Geometry: final body of the model. Coordinates: model frame, mm. Face numbers are marked on the shaded views. A direction names the side the tool comes from. Coordinates: 2 decimals unless noted, no trailing zeros. Write each loop counter-clockwise with the first axis right and the second up, starting at its lowest first coordinate (ties: lowest second). Pieces come first, ordered by that corner, then holes. Notation, with made-up numbers: M -34.75,48.25 L -30.75,48.25 A31 ccw -30.75,78.25 Z; hole C -1.75,17 d1. An arc over 180 degrees is marked long. Write item = value, one per line. Start each with the question number.
Item 1: Reachability of the marked faces 1 and 2 from +Z, -Z, +X, -X, +Y, -Y: full face, straight path, thin tool, end or side. Return the list, or none.
Item 2: Section A-A on y = 5. Output: boundary loops of the cut face in (x, z), plus the area to 3 significant figures.
Item 3: Section C-C on z = 1.25. Output: boundary loops of the cut face in (x, y).
Item 4: First-contact query: pin 1 Ø2 at (x, y) = (9, 2.5) entering from +Z; pin 2 Ø4 at (x, y) = (12, 5) entering from +Z. Flat tips, straight axial feed; report the tip coordinate or a pass-through.
Item 5: Section D-D on y = 7.75. Output: boundary loops of the cut face in (x, z).
Item 6: Section B-B on x = 12. Output: boundary loops of the cut face in (y, z), plus the area to 3 significant figures.
Item 7: Ray query, L1, parallel to Y at x = 12, z = 1.2; L2, parallel to Z at x = 14.25, y = 7; L3, parallel to X at y = 6, z = 0.75. Return the intervals inside material, ascending. Write a range as [from, to].
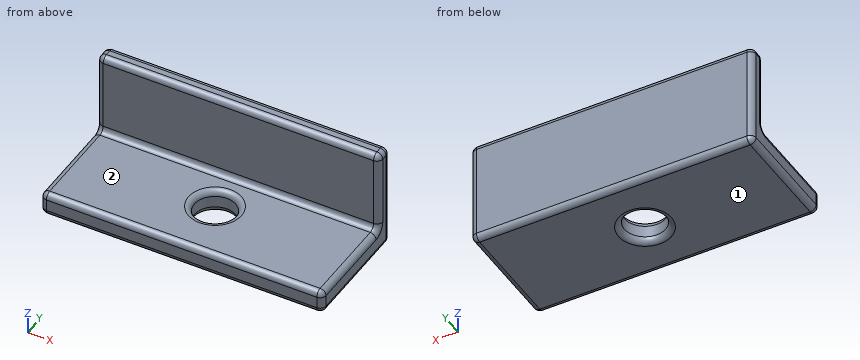
from build123d import *

# Parameters (mm, degrees)
CROQUIS1_W              = 24
CROQUIS1_H              = 10
CROQUIS1_R              = 1.75
SALIENTE_EXTRUIR1_DEPTH = 2
CROQUIS2_W              = 24
CROQUIS2_H              = 1.5
SALIENTE_EXTRUIR2_DEPTH = 7
REDONDEO1_R             = 0.5


with BuildPart() as part:
    # Croquis1 → Saliente-Extruir1 (new body)
    with BuildSketch(Plane.XY):
        with Locations((12, 5)):
            Rectangle(CROQUIS1_W, CROQUIS1_H)
        with Locations((12, 5)):
            Circle(CROQUIS1_R, mode=Mode.SUBTRACT)
    extrude(amount=SALIENTE_EXTRUIR1_DEPTH)

    # Croquis2 → Saliente-Extruir2 (add)
    with BuildSketch(Plane.XY.offset(2)):
        with Locations((12, 9.25)):
            Rectangle(CROQUIS2_W, CROQUIS2_H)
    extrude(amount=SALIENTE_EXTRUIR2_DEPTH)

    # Redondeo1
    redondeo1_edges = [part.edges().sort_by_distance(p)[0] for p in [
        (10.25, 5, 0),
        (10.25, 5, 2),
        (24, 4.25, 2),
        (0, 4.25, 2),
        (24, 8.5, 5.5),
        (12, 8.5, 2),
        (0, 8.5, 5.5),
        (24, 9.25, 9),
        (12, 10, 9),
        (0, 9.25, 9),
        (12, 8.5, 9),
        (12, 10, 0),
        (24, 5, 0),
        (12, 0, 0),
        (0, 5, 0),
        (0, 10, 4.5),
        (24, 10, 4.5),
        (24, 0, 1),
        (0, 0, 1),
        (12, 0, 2),
    ]]
    fillet(redondeo1_edges, radius=REDONDEO1_R)


solid = part.part
Responses:
q1.face_1 = -Z, +X, -X, +Y, -Y
q1.face_2 = +Z, +X, -X, -Y
q2.outline = M 0,0.5 A0.5 ccw 0.5,0 L 9.75,0 A0.5 ccw 10.25,0.5 L 10.25,1.5 A0.5 ccw 9.75,2 L 0.5,2 A0.5 ccw 0,1.5 Z; M 13.75,0.5 A0.5 ccw 14.25,0 L 23.5,0 A0.5 ccw 24,0.5 L 24,1.5 A0.5 ccw 23.5,2 L 14.25,2 A0.5 ccw 13.75,1.5 Z
q2.area = 40.6 mm²
q3.outline = M 0,0.5 A0.5 ccw 0.5,0 L 23.5,0 A0.5 ccw 24,0.5 L 24,9.5 A0.5 ccw 23.5,10 L 0.5,10 A0.5 ccw 0,9.5 Z; hole C 12,5 d3.5
q4.pin_1 = 2
q4.pin_2 = 1.93
q5.outline = M 0,0.5 A0.5 ccw 0.5,0 L 23.5,0 A0.5 ccw 24,0.5 L 24,1.5 A0.5 ccw 23.5,2 L 0.5,2 A0.5 ccw 0,1.5 Z
q6.outline = M 0,0.5 A0.5 ccw 0.5,0 L 2.75,0 A0.5 ccw 3.25,0.5 L 3.25,1.5 A0.5 ccw 2.75,2 L 0.5,2 A0.5 ccw 0,1.5 Z; M 6.75,0.5 A0.5 ccw 7.25,0 L 9.5,0 A0.5 ccw 10,0.5 L 10,8.5 A0.5 ccw 9.5,9 L 9,9 A0.5 ccw 8.5,8.5 L 8.5,2.5 A0.5 cw 8,2 L 7.25,2 A0.5 ccw 6.75,1.5 Z
q6.area = 23.1 mm²
q7.L1 = [0, 3.25], [6.75, 10]
q7.L2 = [0, 2]
q7.L3 = [0, 10.56], [13.44, 24]
